For this review, take the finished solid that the model builds, in its own axes (mm). Face numbers are marked on the shaded views. Round coordinates to 2 decimals unless told otherwise and drop trailing zeros. Order: outer loops, then holes, each group sorted by start corner. A loop starts at its lowest first (then second) coordinate and runs counter-clockwise, first axis right, second up.
```python
from build123d import *

# Parameters (mm, degrees)
EXTRUDE_1_DEPTH      = 3.5
EXTRUDE_1_DEPTH_BACK = 3.5
SKETCH_1_R           = 26
SKETCH_1_R_2         = 20
SKETCH_2_R           = 24
SKETCH_2_R_2         = 22
CUT_EXTRUDE_1_DEPTH  = 1


with BuildPart() as part:
    # 草图1 → 拉伸1 (new, two sides: drawn at the far end of the back side and taken through both)
    with BuildSketch(Plane.XY.offset(-EXTRUDE_1_DEPTH_BACK)):
        Circle(SKETCH_1_R)
        Circle(SKETCH_1_R_2, mode=Mode.SUBTRACT)
    extrude(amount=EXTRUDE_1_DEPTH + EXTRUDE_1_DEPTH_BACK)

    # 草图2 → 切除-拉伸1 (cut)
    with BuildSketch(Plane.XY.offset(3.5)):
        Circle(SKETCH_2_R)
        Circle(SKETCH_2_R_2, mode=Mode.SUBTRACT)
    cut_extrude_1 = extrude(amount=-CUT_EXTRUDE_1_DEPTH, mode=Mode.SUBTRACT)

    # 镜向1: 切除-拉伸1 across plane
    add(cut_extrude_1.mirror(Plane.XY), mode=Mode.SUBTRACT)


solid = part.part
```
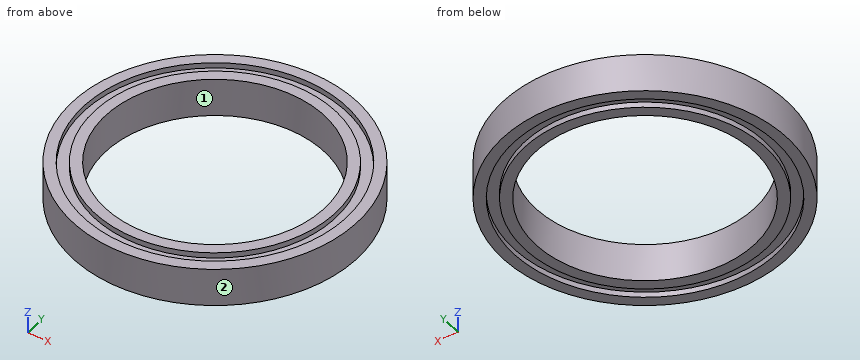
Q1. Take a section at A-A, the plane x = 0. State the section outline as (y, z) points, plus the area to 3 significant figures.
Q2. Take a section at C-C, the plane z = 1.5. State the section outline as (x, y) points.
Q3. Clearance check with flat-ended pins moving along their axes: pin 1 (3 mm diameter, centred on x = 1.5, z = 0.5, fed in from -Y); pin 2 (3 mm diameter, centred on x = 13, z = -1.5, fed in from -Y); pin 3 (6 mm diameter, centred on x = -13.5, y = -10.5, fed in from -Z); pin 4 (3 mm diameter, centred on x = 18, y = 1, fed in from -Z). State where each tip first meets the part, or that it passes through.
Q4. Mouldability with a two-part tool opening along Y and no side actions: class the marked faces 1 and 2 as +Y half, -Y half, draft (parallel to the pull), parting line (faces both ways), or undercut.
Q5. Wall thickness on line 1 (Y direction, x = 0, z = 3.35); line 2 (X direction, y = -10.5, z = 3.25); line 3 (Y direction, x = 0, z = 0.75): over which ranges is each line inside the solid? List them lowest first.
Working result:
1. outline: (-26, -3.5) - (-24, -3.5) - (-24, -2.5) - (-22, -2.5) - (-22, -3.5) - (-20, -3.5) - (-20, 3.5) - (-22, 3.5) - (-22, 2.5) - (-24, 2.5) - (-24, 3.5) - (-26, 3.5) - close; (20, -3.5) - (22, -3.5) - (22, -2.5) - (24, -2.5) - (24, -3.5) - (26, -3.5) - (26, 3.5) - (24, 3.5) - (24, 2.5) - (22, 2.5) - (22, 3.5) - (20, 3.5) - close
1. area: 76.0 mm2
2. outline: circle Ø52 at (0, 0); hole circle Ø40 at (0, 0)
3. pin 1: stops at y = -26
3. pin 2: stops at y = -23.32
3. pin 3: stops at z = -3.5
3. pin 4: passes through
4. face 1: undercut
4. face 2: parting line
5. line 1: y = -26 to -24, -22 to -20, 20 to 22, 24 to 26
5. line 2: x = -23.79 to -21.58, -19.33 to -17.02, 17.02 to 19.33, 21.58 to 23.79
5. line 3: y = -26 to -20, 20 to 26
